Design review of the part built by this model. Coordinates are the model's own, in mm. A direction names the side the tool comes from. Give positions to 0.01 mm unless a question says otherwise; leave off trailing zeros. Write each loop counter-clockwise with the first axis right and the second up, starting at its lowest first coordinate (ties: lowest second). Pieces come first, ordered by that corner, then holes. Notation, with made-up numbers: (68.25, -4) -> (84.25, -4) arc R26 ccw to (84.25, 24) -> close; hole circle Ø4 at (45.5, 35). An arc over 180 degrees is marked (long way). Answer as a JSON object with one key per item and string values.
Autodesk Inventor part; units mm, degrees
ref_plane "YZ Plane" through (0, 0, 0) normal (1, 0, 0) x (0, 1, 0)
ref_plane "XZ Plane" through (0, 0, 0) normal (0, 1, 0) x (-1, 0, 0)
ref_plane "XY Plane" through (0, 0, 0) normal (0, 0, 1) x (1, 0, 0)
sketch "Sketch1" plane through (0, 0, 0) normal (0, 0, 1) x (1, 0, 0)
  circle A0 centre (0, 0) radius 1.621
  dimension "d0" = 3.242
extrude "Extrusion1" add sketch "Sketch1" along normal blind 30
sketch "Sketch2" plane through (0, 0, 30) normal (0, 0, 1) x (1, 0, 0)
  circle A0 centre (0, 0) radius 3
  dimension "d3" = 6
extrude "Extrusion2" add sketch "Sketch2" along normal blind 3
sketch "Sketch3" plane through (0, 0, 33) normal (0, 0, 1) x (1, 0, 0)
  line L0 (1.1547, 2) -> (2.3094, 0)
  line L1 (2.3094, 0) -> (1.1547, -2)
  line L2 (1.1547, -2) -> (-1.1547, -2)
  line L3 (-1.1547, -2) -> (-2.3094, 0)
  line L4 (-2.3094, 0) -> (-1.1547, 2)
  line L5 (-1.1547, 2) -> (1.1547, 2)
  point P0 (0, 0)
  point P1 (0, 0)
  point P2 (0, 2)
  dimension "d7" = 4
  dimension "d9" = 3.4641
extrude "Extrusion3" cut sketch "Sketch3" against normal blind 2
thread "Thread4"
properties part number "M4 union"
(1) For line 1 along Z through (x, y) = (-1.95, -1.9); line 2 along X through (y, z) = (-0.05, 8.5); line 3 along Z through (x, y) = (1.7, -0.85), list the stretches that pass through material, from the lowest coordinate up.
Here are the results:
{"line 1": "z = 30 to 33", "line 2": "x = -1.62 to 1.62", "line 3": "z = 30 to 31"}
(2) Clearance check with flat-ended pins moving along their axes: pin 1 (1 mm diameter, centred on y = 0.5, z = 19, fed in from +X); pin 2 (1 mm diameter, centred on x = -1, y = -0.5, fed in from +Z); pin 3 (3 mm diameter, centred on x = -1.5, z = 21, fed in from -Y). State where each tip first meets the part, or that it passes through.
Here are the results:
{"pin 1": "stops at x = 1.62", "pin 2": "stops at z = 31", "pin 3": "stops at y = -1.62"}
(3) The part is to be moulded in two halves that separate along X. For faces 4 (the cylindrical face through (0.748, 1.438, 14.79)), 5 (the flat face through (2, 1, 33)), 6 (the flat face through (-1.724, -1.014, 32.014)), say which applies: +X half, -X half, draft (parallel to the pull), parting line (faces both ways), or undercut.
Here are the results:
{"face 4": "parting line", "face 5": "draft", "face 6": "undercut"}
(4) We need section A-A, the plane x = -0.55. State the section outline as (y, z) points, then the cut area to 3 significant figures.
Here are the results:
{"outline": "(-2.95, 30) -> (-1.52, 30) -> (-1.52, 0) -> (1.52, 0) -> (1.52, 30) -> (2.95, 30) -> (2.95, 33) -> (2, 33) -> (2, 31) -> (-2, 31) -> (-2, 33) -> (-2.95, 33) -> close", "area": "101 mm²"}
(5) We need section C-C, the plane z = 30.5. State the section outline as (x, y) points.
Here are the results:
{"outline": "circle Ø6 at (0, 0)"}
(6) We need section D-D, the plane x = 2. State the section outline as (y, z) points, then the cut area to 3 significant figures.
Here are the results:
{"outline": "(-2.24, 30) -> (2.24, 30) -> (2.24, 33) -> (0.54, 33) -> (0.54, 31) -> (-0.54, 31) -> (-0.54, 33) -> (-2.24, 33) -> close", "area": "11.3 mm²"}
(7) For faces 1 (the flat face through (1.74, -0.99, 32.01)), 2 (the cylindrical face through (-3, 0, 31)), 3 (the flat face through (1.3, -1.3, 30)), list the 3-axis set-ups (+Z, -Z, +X, -X, +Y, -Y) from which the entire face can be reached by the end or side of a thin tool; tool diameter is ignored.
Here are the results:
{"face 1": "+Z", "face 2": "+Z, -Z", "face 3": "-Z"}
(8) We need section B-B, the plane y = -1.25. State the section outline as (x, z) points, then the cut area to 3 significant figures.
Here are the results:
{"outline": "(-2.73, 30) -> (-1.03, 30) -> (-1.03, 0) -> (1.03, 0) -> (1.03, 30) -> (2.73, 30) -> (2.73, 33) -> (1.59, 33) -> (1.59, 31) -> (-1.59, 31) -> (-1.59, 33) -> (-2.73, 33) -> close", "area": "71.9 mm²"}
